Can you work these out from the model? Positions are in its coordinate system, mm. A direction names the side the tool comes from. Coordinates: 2 decimals unless noted, no trailing zeros. Write each loop counter-clockwise with the first axis right and the second up, starting at its lowest first coordinate (ties: lowest second). Pieces come first, ordered by that corner, then holes. Notation, with made-up numbers: (45, 28) -> (50, 28) arc R12 cw to (50, 35) -> close; hole circle Ø9 at (-2.75, 19). An arc over 180 degrees is marked (long way). Use one line per item in the form item = value.
Autodesk Inventor part; units mm, degrees
ref_plane "YZ Plane" through (0, 0, 0) normal (1, 0, 0) x (0, 1, 0)
ref_plane "XZ Plane" through (0, 0, 0) normal (0, 1, 0) x (-1, 0, 0)
ref_plane "XY Plane" through (0, 0, 0) normal (0, 0, 1) x (1, 0, 0)
sketch "Skizze1" plane through (0, 0, 0) normal (0, 0, 1) x (1, 0, 0)
  line L0 (-5, 5) -> (5, 5)
  line L1 (5, 5) -> (5, -5)
  line L2 (5, -5) -> (-5, -5)
  line L3 (-5, -5) -> (-5, 5)
  point P0 (0, 0)
  point P1 (5, 0)
  point P2 (0, -5)
  dimension "d0" = 10
  dimension "d1" = 10
extrude "Extrusion1" add sketch "Skizze1" along normal blind 10
sketch "Skizze2" plane through (0, 0, 10) normal (0, 0, 1) x (1, 0, 0)
  circle A0 centre (0, 0) radius 3.75
  dimension "d4" = 7.5
extrude "Extrusion2" add sketch "Skizze2" along normal blind 1.76
fillet "Rundung1" radius 0.25 1 edges at (-3.75, 0, 11.76)
sketch "Skizze3" plane through (0, 0, 11.76) normal (0, 0, 1) x (1, 0, 0)
  circle A0 centre (0, 0) radius 3.5
  circle A1 centre (0, 0) radius 2.25
  dimension "d8" = 4.5
extrude "Extrusion3" add sketch "Skizze3" along normal blind 0.5 contours A1
sketch "Skizze4" plane through (0, 0, 12.26) normal (0, 0, 1) x (1, 0, 0)
  circle A0 centre (0, 0) radius 2.25
  circle A1 centre (0, 0) radius 3.5
  dimension "d11" = 7
extrude "Extrusion4" add sketch "Skizze4" along normal blind 7.6 contours A0 | A1
fillet "Rundung2" radius 0.25 1 edges at (-3.5, 0, 19.86)
fillet "Rundung3" radius 0.1 12 edges at (-5, -5, 5) (-5, 5, 5) (-5, 0, 10) (0, -5, 10) (5, 0, 10) (5, -5, 5) (0, -5, 0) (-5, 0, 0) (0, 5, 0) (0, 5, 10) (5, 5, 5) (5, 0, 0)
sketch "Skizze5" plane through (-4.9, 5, 0.1) normal (0, 1, 0) x (1, 0, 0)
  point P0 (4.9, 0.1)
  point P1 (4.9, -1.1417)
hole "Hole2" at (0, 5, 1.2417) direction (0, -1, 0) diameter 2 depth 5 tip angle 118
properties part number "Taster"
Q1. Will these pins go through, and if not, where does the flat tip stop? pin 1 (3 mm diameter, centred on x = -2, y = -3, fed in from +Z); pin 2 (1 mm diameter, centred on y = 3, z = 16.5, fed in from +X).
Return value:
pin_1 = 19.86
pin_2 = 2.45
Q2. Suppose I cut it at A-A (x = 4). Write out the boundary of the cut face in (y, z).
Return value:
outline = (-5, 0.1) arc R0.1 ccw to (-4.9, 0) -> (4.9, 0) arc R0.1 ccw to (5, 0.1) -> (5, 9.9) arc R0.1 ccw to (4.9, 10) -> (-4.9, 10) arc R0.1 ccw to (-5, 9.9) -> close
Q3. For faces 1 (the flat face through (0, 5, 5)), 2 (the flat face through (-2.2, 3.3, 10)), 3 (the flat face through (2.3, -0.7, 11.76)), which set-ups out of +Z, -Z, +X, -X, +Y, -Y let a thin tool reach every point of the face, with its end or its side?
Return value:
face_1 = +Z, -Z, +X, -X, +Y
face_2 = +Z
face_3 = none
Q4. If I drill on line 1 (Z direction, x = 0, y = 1.4); line 2 (Z direction, x = 0, y = 3.4); line 3 (Z direction, x = 0, y = 3.9), over which ranges is the centre line in solid material (lowest first)? Write a range as from..to.
Return value:
line_1 = 0..0.24, 2.24..19.86
line_2 = 0..0.24, 2.24..11.76, 12.26..19.81
line_3 = 0..0.24, 2.24..10
Q5. Thinking about a two-plate mould opening in Z: for faces 4 (the cylindrical face through (0.61, 2.46, 0.45)), 5 (the flat face through (-5, 0, 5)), 6 (the flat face through (0, 0, 19.86)), which applies, released by +Z, released by -Z, zero draft, split by the parting line, or undercut?
Return value:
face_4 = undercut
face_5 = zero draft
face_6 = released by +Z
Q6. Suppose I cut it at B-B (z = 13.25). Write out the boundary of the cut face in (x, y), then the cut area to 3 significant figures.
Return value:
outline = circle Ø7 at (0, 0)
area = 38.5 mm2
